```python
from build123d import *

# Parameters (mm, degrees)
BODY_DEPTH               = 24
SKETCH2_W                = 6
SKETCH2_H                = 5
FIXATION_CUTOUT_DEPTH    = 107.733312513
FIXATION_CUTOUT_ROUNDS_R = 2.5


with BuildPart() as part:
    # Sketch1 → body (new body)
    with BuildSketch(Plane.XY):
        Polygon((0, 0), (96, 0), (96, 2), (84, 2), (84, 42), (12, 42), (12, 2), (0, 2), align=None)
    extrude(amount=BODY_DEPTH)

    # Sketch2 → fixation_cutout (cut, through all)
    with BuildSketch(Plane(origin=(0, 2, 0), x_dir=(1, 0, 0), z_dir=(0, 1, 0))):
        with Locations((3, -9.5)):
            Rectangle(SKETCH2_W, SKETCH2_H)
        with Locations((93, -9.5)):
            Rectangle(SKETCH2_W, SKETCH2_H)
    extrude(amount=-FIXATION_CUTOUT_DEPTH, mode=Mode.SUBTRACT)

    # fixation_cutout_rounds
    fixation_cutout_rounds_edges = [part.edges().sort_by_distance(p)[0] for p in [
        (90, 1, 12),
        (90, 1, 7),
        (6, 1, 12),
        (6, 1, 7),
    ]]
    fillet(fixation_cutout_rounds_edges, radius=FIXATION_CUTOUT_ROUNDS_R - 0.0001)  # a hair under: the kernel refuses the full size


solid = part.part
```
Geometry: final body of the model. Coordinates: model frame, mm. A direction names the side the tool comes from. Round coordinates to 2 decimals unless told otherwise and drop trailing zeros. Order: outer loops, then holes, each group sorted by start corner. A loop starts at its lowest first (then second) coordinate and runs counter-clockwise, first axis right, second up. Notation, with made-up numbers: M -20.75,-13 L 23.25,-13 A13 ccw 23.25,3 Z; hole C 29,-2 d9. An arc over 180 degrees is marked long. One line per item, written item: value.
(1) Pin query (flat end, axial travel): P1, Ø10, axis at y = 32.5, z = 5, coming from the -X side; P2, Ø12, axis at x = 41.5, y = 18.5, coming from the -Z side; P3, Ø6, axis at x = 89, z = 6, coming from the +Y side; P4, Ø1.5, axis at y = 22, z = 19, coming from the +X side. Return the tip coordinate at first contact, or that it passes through.
Result sheet:
P1: x = 12
P2: z = 0
P3: y = 2
P4: x = 84
(2) Cut plane A-A (z = 3.75). Return the cut outline in (x, y), and give its area (3 significant figures).
Result sheet:
outline: M 0,0 L 96,0 L 96,2 L 84,2 L 84,42 L 12,42 L 12,2 L 0,2 Z
area: 3,070 mm2
(3) Cut plane D-D (z = 11). Return the cut outline in (x, y).
Result sheet:
outline: M 5.5,0 L 90.5,0 L 90.5,2 L 84,2 L 84,42 L 12,42 L 12,2 L 5.5,2 Z
(4) Cut plane C-C (x = 8.5). Return the cut outline in (y, z).
Result sheet:
outline: M 0,0 L 2,0 L 2,24 L 0,24 Z
(5) Line query: probe 1 along X at (y, z) = (6, 1.75); probe 2 along Y at (x, z) = (11.5, 12). Output: solid intervals per line, ascending. Write a range as [from, to].
Result sheet:
probe 1: [12, 84]
probe 2: [0, 2]
(6) Reachability of faces 1 (the flat face through (12, 22, 12)), 2 (the cylindrical face through (90.713, 0.986, 11.248)), 3 (the flat face through (2, 1, 12)) from +Z, -Z, +X, -X, +Y, -Y: full face, straight path, thin tool, end or side. Return the list, or none.
Result sheet:
face 1: +Z, -Z, -X, +Y
face 2: +X, +Y, -Y
face 3: -X, +Y, -Y
(7) Cut plane B-B (y = 20). Return the cut outline in (x, z), and give its area (3 significant figures).
Result sheet:
outline: M 12,0 L 84,0 L 84,24 L 12,24 Z
area: 1,730 mm2
(8) Pull-direction query (Z, two-part tool) for faces 4 (the flat face through (96, 1, 18)), 5 (the flat face through (47, 21, 24)), 6 (the flat face through (94, 1, 7)); classes: pulls with the +Z half, pulls with the -Z half, needs draft (parallel to the pull), parting line crosses it, or undercut.
Result sheet:
face 4: needs draft
face 5: pulls with the +Z half
face 6: undercut
